Solid Edge part; units mm, degrees
sketch "Sketch1" plane through (0, 0, 0) normal (0, -1, 0) x (1, 0, 0)
  line L0 (40.5, -5) -> (-40.5, -5)
  line L1 (-40.5, -5) -> (-40.5, 5)
  line L2 (-40.5, 5) -> (40.5, 5)
  line L3 (40.5, 5) -> (40.5, -5)
  dimension "D1" = 40.5
  dimension "D2" = 40.5
extrude "Protrusion1" add sketch "Sketch1" against normal blind 42.8
hole "Agujero_1" at (-16.5, 0, 0) direction (0, 1, 0) diameter 6.5 end through all
hole "Hole1" at (30.5, 0, 0) direction (0, 1, 0) diameter 6.5 end through all
sketch "Sketch2" plane through (0, 21.4, -5) normal (0, 0, -1) x (1, 0, 0)
  line L0 (24.5, -3.6) -> (24.5, 21.4)
  line L1 (4.5, -3.6) -> (24.5, -3.6)
  line L2 (4.5, -3.6) -> (4.5, 21.4)
  dimension "D1" = 4.5
  dimension "D2" = 24.5
extrude "Cutout1" cut sketch "Sketch2" against normal through all material side at (24.45, 12.5, -5)
properties part number "1976-1100-016" material "Aluminio, 7075-T6"
Could you check a few things on this model? Use its own coordinates, in mm. A direction names the side the tool comes from. Round coordinates to 2 decimals unless told otherwise and drop trailing zeros. Loops run counter-clockwise (first coordinate to the right, second up) from the corner with the lowest first, then second, coordinate; pieces in that order, holes last. Notation, with made-up numbers: (51, 1.5) - (105, 1.5) arc R27 cw to (105, 27.5) - close; hole circle Ø2 at (17.5, 60). An arc over 180 degrees is marked (long way). Answer as CSV lines item,"result".
1. I want a section at B-B on z = 0. List the corners of the cut face in (x, y) for me.
Filled in:
outline,"(-40.5, 0) - (-19.75, 0) - (-19.75, 42.8) - (-40.5, 42.8) - close; (-13.25, 0) - (4.5, 0) - (4.5, 25) - (24.5, 25) - (24.5, 0) - (27.25, 0) - (27.25, 42.8) - (-13.25, 42.8) - close; (33.75, 0) - (40.5, 0) - (40.5, 42.8) - (33.75, 42.8) - close"
2. On a 3-axis mill with a long thin cutter (end or side, diameter ignored), from which of +Z, -Z, +X, -X, +Y, -Y can I reach the whole of each face in a straight line? I mean faces 1 (the face through (-1, 21, 5)), 2 (the face through (24.5, 13, 0)). Say none if no direction works.
Filled in:
face 1,"+Z, +X, -X, +Y, -Y"
face 2,"+Z, -Z, -Y"
3. Please list where these lines run through material, in increasing order: line 1 along X through (y, z) = (28, 0); line 2 along X through (y, z) = (13, 0); line 3 along X through (y, z) = (14.5, 4.25). Write a range as [from, to].
Filled in:
line 1,"x = [-40.5, -19.75], [-13.25, 27.25], [33.75, 40.5]"
line 2,"x = [-40.5, -19.75], [-13.25, 4.5], [24.5, 27.25], [33.75, 40.5]"
line 3,"x = [-40.5, 4.5], [24.5, 40.5]"
4. I want a section at A-A on y = 10.5. List the corners of the cut face in (x, z) for me.
Filled in:
outline,"(-40.5, -5) - (4.5, -5) - (4.5, 5) - (-40.5, 5) - close; (24.5, -5) - (40.5, -5) - (40.5, 5) - (24.5, 5) - close; hole circle Ø6.5 at (-16.5, 0); hole circle Ø6.5 at (30.5, 0)"
5. I want a section at D-D on y = 35. List the corners of the cut face in (x, z) for me, then the cut area to 3 significant figures.
Filled in:
outline,"(-40.5, -5) - (40.5, -5) - (40.5, 5) - (-40.5, 5) - close; hole circle Ø6.5 at (-16.5, 0); hole circle Ø6.5 at (30.5, 0)"
area,"744 mm^2"
6. I want a section at C-C on x = -16.5. List the corners of the cut face in (y, z) for me.
Filled in:
outline,"(0, -5) - (42.8, -5) - (42.8, -3.25) - (0, -3.25) - close; (0, 3.25) - (42.8, 3.25) - (42.8, 5) - (0, 5) - close"
7. For pin 1 Ø4 at (x, z) = (-16.5, 0) entering from +Y; pin 2 Ø1.5 at (x, z) = (13, 3) entering from -Y, each with a flat end and sliding along its axis, tell me the tip position at first contact or that it passes through.
Filled in:
pin 1,"passes through"
pin 2,"stops at y = 25"
8. We'd pull the mould along Z, two halves only. Please class faces 3 (the face through (34, 0, 0)), 4 (the face through (1, 21, -5)), 5 (the face through (-13.278, 21.1, 0.423)): +Z half, -Z half, draft (parallel to the pull), parting line (faces both ways), or undercut.
Filled in:
face 3,"draft"
face 4,"-Z half"
face 5,"undercut"
